from build123d import *

# Parameters (mm, degrees)
SKETCH1_W           = 279.4
SKETCH1_H           = 101.6
BOSS_EXTRUDE1_DEPTH = 101.6
SKETCH2_W           = 279.4
SKETCH2_H           = 50.868063328
CUT_EXTRUDE1_DEPTH  = 50.8
SKETCH3_R           = 12.7
CUT_EXTRUDE5_DEPTH  = 50.8
SKETCH7_R           = 19.05
CUT_EXTRUDE6_DEPTH  = 19.05
SKETCH8_R           = 12.7
CUT_EXTRUDE7_DEPTH  = 76.2
FILLET3_R           = 6.35
CHAMFER3_SIZE       = 6.35


with BuildPart() as part:
    # Sketch1 → Boss-Extrude1 (new body)
    with BuildSketch(Plane.XY):
        with Locations((139.7, 50.8)):
            Rectangle(SKETCH1_W, SKETCH1_H)
    extrude(amount=BOSS_EXTRUDE1_DEPTH)

    # Sketch2 → Cut-Extrude1 (cut)
    with BuildSketch(Plane(origin=(0, 101.6, 0), x_dir=(1, 0, 0), z_dir=(0, 1, 0))):
        with Locations((139.7, -50.8)):
            Rectangle(SKETCH2_W, SKETCH2_H)
    extrude(amount=-CUT_EXTRUDE1_DEPTH, mode=Mode.SUBTRACT)

    # Sketch3 → Cut-Extrude5 (cut)
    with BuildSketch(Plane(origin=(0, 50.8, 0), x_dir=(1, 0, 0), z_dir=(0, 1, 0))):
        with Locations(Location((38.1, -50.8, 0), (0, 0, 270))):
            Circle(SKETCH3_R)
        with Locations(Location((88.9, -50.8, 0), (0, 0, 270))):
            Circle(SKETCH3_R)
        with Locations(Location((190.5, -50.8, 0), (0, 0, 270))):
            Circle(SKETCH3_R)
        with Locations(Location((241.3, -50.8, 0), (0, 0, 270))):
            Circle(SKETCH3_R)
    extrude(amount=-CUT_EXTRUDE5_DEPTH, mode=Mode.SUBTRACT)

    # Sketch7 → Cut-Extrude6 (cut)
    with BuildSketch(Plane(origin=(0, 50.8, 0), x_dir=(1, 0, 0), z_dir=(0, 1, 0))):
        with Locations(Location((139.7, -50.8, 0), (0, 0, 270))):
            Circle(SKETCH7_R)
    extrude(amount=-CUT_EXTRUDE6_DEPTH, mode=Mode.SUBTRACT)

    # Sketch8 → Cut-Extrude7 (cut)
    with BuildSketch(Plane(origin=(0, 31.75, 0), x_dir=(1, 0, 0), z_dir=(0, 1, 0))):
        with Locations(Location((139.7, -50.8, 0), (0, 0, 270))):
            Circle(SKETCH8_R)
    extrude(amount=-CUT_EXTRUDE7_DEPTH, mode=Mode.SUBTRACT)

    # Fillet3
    fillet3_edges = [part.edges().sort_by_distance(p)[0] for p in [
        (38.1, 50.8, 38.1),
        (88.9, 50.8, 38.1),
    ]]
    fillet(fillet3_edges, radius=FILLET3_R)

    # Chamfer3
    chamfer3_edges = [part.edges().sort_by_distance(p)[0] for p in [
        (190.5, 50.8, 38.1),
        (241.3, 50.8, 38.1),
    ]]
    chamfer(chamfer3_edges, length=CHAMFER3_SIZE)


solid = part.part
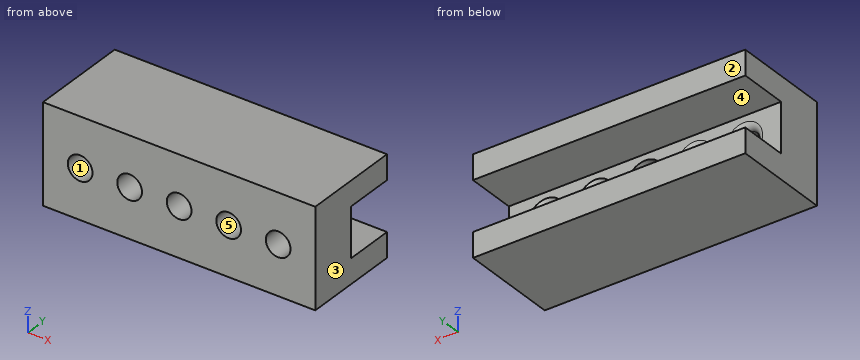
Design review of the part built by this model. Coordinates are the model's own, in mm. Face numbers are marked on the shaded views. A direction names the side the tool comes from. Round coordinates to 2 decimals unless told otherwise and drop trailing zeros. Write each loop counter-clockwise with the first axis right and the second up, starting at its lowest first coordinate (ties: lowest second). Pieces come first, ordered by that corner, then holes.
Item 1: Consider section B-B on y = 68.5. Give the boundary of the cut face in (x, z).
Item 2: For the marked faces 4 and 5, list the 3-axis set-ups (+Z, -Z, +X, -X, +Y, -Y) from which the entire face can be reached by the end or side of a thin tool; tool diameter is ignored.
Item 3: Consider section D-D on x = 241.3. Give the boundary of the cut face in (y, z).
Item 4: For pin 1 Ø20.5 at (x, z) = (241.3, 50.8) entering from +Y; pin 2 Ø19 at (x, z) = (142, 44) entering from +Y, all flat-tipped, find the tip position at first contact; note any pin that passes through.
Item 5: Consider section A-A on x = 88.9. Give the boundary of the cut face in (y, z).
Item 6: Wall thickness on L1, parallel to X at y = 32, z = 50.8; L2, parallel to X at y = 11, z = 50.8; L3, parallel to Z at x = 213.5, y = 96: over which ranges is each line inside the solid? List them lowest first.
Item 7: Consider section C-C on y = 39.5. Give the boundary of the cut face in (x, z), and give its area (3 significant figures).
Item 8: Draft analysis for pull direction X (two halves, no side actions). For the marked faces 1, 2 and 3, state which applies: released by +X, released by -X, zero draft, split by the parting line, or undercut.
Check values:
1. outline: (0, 0) - (279.4, 0) - (279.4, 25.37) - (0, 25.37) - close; (0, 76.23) - (279.4, 76.23) - (279.4, 101.6) - (0, 101.6) - close
2. face 4: +X, -X, +Y
2. face 5: +Y, -Y
3. outline: (0, 0) - (101.6, 0) - (101.6, 25.37) - (50.8, 25.37) - (50.8, 31.75) - (44.45, 38.1) - (0, 38.1) - close; (0, 63.5) - (44.45, 63.5) - (50.8, 69.85) - (50.8, 76.23) - (101.6, 76.23) - (101.6, 101.6) - (0, 101.6) - close
4. pin 1: passes through
4. pin 2: stops at y = 31.75
5. outline: (0, 0) - (101.6, 0) - (101.6, 25.37) - (50.8, 25.37) - (50.8, 31.75) arc R6.35 ccw to (44.45, 38.1) - (0, 38.1) - close; (0, 63.5) - (44.45, 63.5) arc R6.35 ccw to (50.8, 69.85) - (50.8, 76.23) - (101.6, 76.23) - (101.6, 101.6) - (0, 101.6) - close
6. L1: x = 0 to 25.4, 50.8 to 76.2, 101.6 to 120.65, 158.75 to 177.8, 203.2 to 228.6, 254 to 279.4
6. L2: x = 0 to 25.4, 50.8 to 76.2, 101.6 to 127, 152.4 to 177.8, 203.2 to 228.6, 254 to 279.4
6. L3: z = 0 to 25.37, 76.23 to 101.6
7. outline: (0, 0) - (279.4, 0) - (279.4, 101.6) - (0, 101.6) - close; hole circle Ø25.4 at (38.1, 50.8); hole circle Ø25.4 at (88.9, 50.8); hole circle Ø38.1 at (139.7, 50.8); hole circle Ø25.4 at (190.5, 50.8); hole circle Ø25.4 at (241.3, 50.8)
7. area: 25,200 mm2
8. face 1: undercut
8. face 2: zero draft
8. face 3: released by +X
